```python
from build123d import *

# Parameters (mm, degrees)
SKETCH1_W               = 10
SKETCH1_H               = 10
SKETCH1_W_2             = 7
SKETCH1_H_2             = 7
EXTRUDE_THIN1_DEPTH     = 220
SKETCH2_R               = 2.25
CUT_EXTRUDE1_DEPTH      = 6
CUT_EXTRUDE1_DEPTH_BACK = 6
FILLET1_R               = 0.2


with BuildPart() as part:
    # Sketch1 → Extrude-Thin1 (new body)
    with BuildSketch(Plane(origin=(0, 0, 0), x_dir=(1, 0, 0), z_dir=(0, 1, 0))):
        Rectangle(SKETCH1_W, SKETCH1_H)
        Rectangle(SKETCH1_W_2, SKETCH1_H_2, mode=Mode.SUBTRACT)
    extrude(amount=EXTRUDE_THIN1_DEPTH)

    # Sketch2 → Cut-Extrude1 (cut, two sides)
    with BuildSketch(Plane(origin=(0, 0, 0), x_dir=(0, 0, -1), z_dir=(1, 0, 0))) as cut_extrude1_sk:
        with Locations((0, 215)):
            Circle(SKETCH2_R)
        with Locations((0, 5)):
            Circle(SKETCH2_R)
    extrude(amount=CUT_EXTRUDE1_DEPTH, mode=Mode.SUBTRACT)
    extrude(cut_extrude1_sk.sketch, amount=-CUT_EXTRUDE1_DEPTH_BACK, mode=Mode.SUBTRACT)

    # Fillet1
    fillet1_edges = [part.edges().sort_by_distance(p)[0] for p in [
        (-5, 110, -5),
        (5, 110, -5),
        (5, 110, 5),
        (-5, 110, 5),
    ]]
    fillet(fillet1_edges, radius=FILLET1_R)


solid = part.part
```
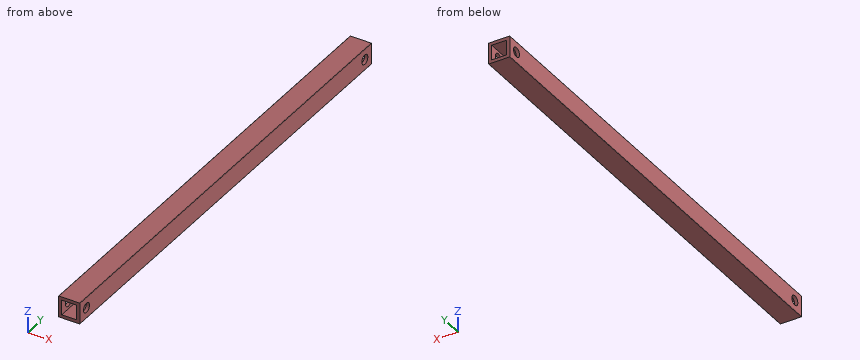
Check sheet for the modelled part. Datum: model origin and axes. Units: mm. Give positions to 0.01 mm unless a question says otherwise; leave off trailing zeros. Write each loop counter-clockwise with the first axis right and the second up, starting at its lowest first coordinate (ties: lowest second). Pieces come first, ordered by that corner, then holes.
Item 1: Cross-section at C-C (y = 215). Enter the section's corners in (x, z), and give its area (3 significant figures).
Item 2: Cross-section at D-D (y = 136). Enter the section's corners in (x, z).
Item 3: Cross-section at A-A (x = -1.25). Enter the section's corners in (y, z).
Item 4: Scan lines: L1, parallel to Y at x = 4.3, z = 0; L2, parallel to Z at x = -2.75, y = 112.5. Record each from-to range of solid material in increasing order.
Item 5: Cross-section at B-B (z = 0). Enter the section's corners in (x, y), and give its area (3 significant figures).
Report:
1. outline: (-5, -4.8) arc R0.2 ccw to (-4.8, -5) - (4.8, -5) arc R0.2 ccw to (5, -4.8) - (5, -2.25) - (3.5, -2.25) - (3.5, -3.5) - (-3.5, -3.5) - (-3.5, -2.25) - (-5, -2.25) - close; (-5, 2.25) - (-3.5, 2.25) - (-3.5, 3.5) - (3.5, 3.5) - (3.5, 2.25) - (5, 2.25) - (5, 4.8) arc R0.2 ccw to (4.8, 5) - (-4.8, 5) arc R0.2 ccw to (-5, 4.8) - close
1. area: 37.5 mm2
2. outline: (-5, -4.8) arc R0.2 ccw to (-4.8, -5) - (4.8, -5) arc R0.2 ccw to (5, -4.8) - (5, 4.8) arc R0.2 ccw to (4.8, 5) - (-4.8, 5) arc R0.2 ccw to (-5, 4.8) - close; hole (-3.5, -3.5) - (3.5, -3.5) - (3.5, 3.5) - (-3.5, 3.5) - close
3. outline: (0, -5) - (220, -5) - (220, -3.5) - (0, -3.5) - close; (0, 3.5) - (220, 3.5) - (220, 5) - (0, 5) - close
4. L1: y = 0 to 2.75, 7.25 to 212.75, 217.25 to 220
4. L2: z = -5 to -3.5, 3.5 to 5
5. outline: (-5, 0) - (-3.5, 0) - (-3.5, 2.75) - (-5, 2.75) - close; (-5, 7.25) - (-3.5, 7.25) - (-3.5, 212.75) - (-5, 212.75) - close; (-5, 217.25) - (-3.5, 217.25) - (-3.5, 220) - (-5, 220) - close; (3.5, 0) - (5, 0) - (5, 2.75) - (3.5, 2.75) - close; (3.5, 7.25) - (5, 7.25) - (5, 212.75) - (3.5, 212.75) - close; (3.5, 217.25) - (5, 217.25) - (5, 220) - (3.5, 220) - close
5. area: 633 mm2
